Work out the finished part from the listing and answer in its coordinate system (mm). A direction names the side the tool comes from. Coordinates: 2 decimals unless noted, no trailing zeros. Order: outer loops, then holes, each group sorted by start corner. A loop starts at its lowest first (then second) coordinate and runs counter-clockwise, first axis right, second up. Notation, with made-up numbers: (51.25, 17.5) -> (94.25, 17.5) arc R19 ccw to (94.25, 28.5) -> close; hole circle Ø11 at (37.25, -9). An arc over 180 degrees is marked (long way). Answer as CSV lines item,"result". Start each with the question number.
Item 1: Section D-D (z = -8.5) is taken. Write down the section's boundary in (x, y).
Item 2: Straight lines are drawn through the part: L1, parallel to X at y = 2.4, z = -17; L2, parallel to X at y = 2.3, z = -7. For each, find the intervals that lie inside material, in ascending order.
Item 3: Which of the six approach directions +Z, -Z, +X, -X, +Y, -Y give full straight-line access (tool end or side, diameter ignored) to faces 5 (the face through (-2, 1, -15)), 6 (the face through (48, 1, -2)), 7 (the face through (45, 1, -10))?
Item 4: For a pull along X with two mould halves and no side action, classify faces 1 (the face through (11.11, 1.48, -4.04)), 2 (the face through (22, 1, 0)), 3 (the face through (33.84, 1.48, -16.46)), 4 (the face through (0, 1, -10)) as pulls with the +X half, pulls with the -X half, needs draft (parallel to the pull), parting line crosses it, or undercut.
Item 5: Section C-C (x = 12) is taken. Write down the section's boundary in (y, z), then the cut area to 3 significant figures.
Item 6: This flat-tipped pin is pushed along its axis until it touches: pin 1 Ø1.5 at (x, y) = (15, 2) entering from +Z. Where does it stop, or does it pass through?
Item 7: Section A-A (z = -4.5) is taken. Write down the section's boundary in (x, y), then the cut area to 3 significant figures.
Item 8: Section B-B (y = 1.9) is taken. Write down the section's boundary in (x, z).
```python
from build123d import *

# Parameters (mm, degrees)
SKETCH1_W           = 3
SKETCH1_H           = 5
SKETCH1_R           = 1
BOSS_EXTRUDE1_DEPTH = 3


with BuildPart() as part:
    # Sketch1 → Boss-Extrude1 (new body)
    # profile 1 of 6: a face of its own
    with BuildSketch(Plane(origin=(0, 0, 0), x_dir=(1, 0, 0), z_dir=(0, 1, 0))):
        with Locations((-1.5, 17.5)):
            Rectangle(SKETCH1_W, SKETCH1_H)
    # profile 2 of 6: a face of its own
    with BuildSketch(Plane(origin=(0, 0, 0), x_dir=(1, 0, 0), z_dir=(0, 1, 0))):
        Polygon((22.5, 0), (22.5, 20), (0, 20), (0, 15), (0, 5), (0, 0), align=None)
        with Locations(Location((12, 4.5, 0), (0, 0, 270))):
            Circle(SKETCH1_R, mode=Mode.SUBTRACT)
        with Locations(Location((12, 17, 0), (0, 0, 270))):
            Circle(SKETCH1_R, mode=Mode.SUBTRACT)
    # profile 3 of 6: a face of its own
    with BuildSketch(Plane(origin=(0, 0, 0), x_dir=(1, 0, 0), z_dir=(0, 1, 0))):
        Polygon((45, 20), (22.5, 20), (22.5, 0), (45, 0), (45, 5), (45, 15), align=None)
        with Locations(Location((33, 4.5, 0), (0, 0, 270))):
            Circle(SKETCH1_R, mode=Mode.SUBTRACT)
        with Locations(Location((33, 17, 0), (0, 0, 270))):
            Circle(SKETCH1_R, mode=Mode.SUBTRACT)
    # profile 4 of 6: a face of its own
    with BuildSketch(Plane(origin=(0, 0, 0), x_dir=(1, 0, 0), z_dir=(0, 1, 0))):
        with Locations((46.5, 17.5)):
            Rectangle(SKETCH1_W, SKETCH1_H)
    # profile 5 of 6: a face of its own
    with BuildSketch(Plane(origin=(0, 0, 0), x_dir=(1, 0, 0), z_dir=(0, 1, 0))):
        with Locations((-1.5, 2.5)):
            Rectangle(SKETCH1_W, SKETCH1_H)
    # profile 6 of 6: a face of its own
    with BuildSketch(Plane(origin=(0, 0, 0), x_dir=(1, 0, 0), z_dir=(0, 1, 0))):
        with Locations((46.5, 2.5)):
            Rectangle(SKETCH1_W, SKETCH1_H)
    extrude(amount=BOSS_EXTRUDE1_DEPTH)


solid = part.part
```
Checked values:
1,outline,"(0, 0) -> (45, 0) -> (45, 3) -> (0, 3) -> close"
2,L1,"x = -3 to 11, 13 to 32, 34 to 48"
2,L2,"x = 0 to 45"
3,face 5,"-X, +Y, -Y"
3,face 6,"+Z, -Z, +X, +Y, -Y"
3,face 7,"+X, +Y, -Y"
4,face 1,"undercut"
4,face 2,"needs draft"
4,face 3,"undercut"
4,face 4,"pulls with the -X half"
5,outline,"(0, -20) -> (3, -20) -> (3, -18) -> (0, -18) -> close; (0, -16) -> (3, -16) -> (3, -5.5) -> (0, -5.5) -> close; (0, -3.5) -> (3, -3.5) -> (3, 0) -> (0, 0) -> close"
5,area,"48.0 mm^2"
6,pin 1,"stops at z = 0"
7,outline,"(-3, 0) -> (11, 0) -> (11, 3) -> (-3, 3) -> close; (13, 0) -> (32, 0) -> (32, 3) -> (13, 3) -> close; (34, 0) -> (48, 0) -> (48, 3) -> (34, 3) -> close"
7,area,"141 mm^2"
8,outline,"(-3, -20) -> (48, -20) -> (48, -15) -> (45, -15) -> (45, -5) -> (48, -5) -> (48, 0) -> (-3, 0) -> (-3, -5) -> (0, -5) -> (0, -15) -> (-3, -15) -> close; hole circle Ø2 at (12, -17); hole circle Ø2 at (12, -4.5); hole circle Ø2 at (33, -17); hole circle Ø2 at (33, -4.5)"
